from build123d import *

# Parameters (mm, degrees)
SKETCH_1_R          = 4
SKETCH_1_R_2        = 2.95
EXTRUDE_1_DEPTH     = 4.5
SKETCH_1_3_R        = 2.95
SKETCH_1_3_R_2      = 2.5
SKETCH_1_3_R_3      = 1.1
EXTRUDE_2_DEPTH     = 1.7
SKETCH_1_4_R        = 2.95
SKETCH_1_4_R_2      = 2.5
SKETCH_1_4_R_3      = 1.1
CUT_EXTRUDE_1_DEPTH = 0.4
SKETCH_2_R          = 0.6
EXTRUDE_3_DEPTH     = 1.7


with BuildPart() as part:
    # Sketch 1 → Extrude 1 (new body)
    with BuildSketch(Plane.XY):
        Circle(SKETCH_1_R)
        Circle(SKETCH_1_R_2, mode=Mode.SUBTRACT)
    extrude(amount=EXTRUDE_1_DEPTH)

    # Sketch 1_3 → Extrude 2 (add)
    # profile 1 of 2: a face of its own
    with BuildSketch(Plane.XY):
        Circle(SKETCH_1_3_R)
        Circle(SKETCH_1_3_R_2, mode=Mode.SUBTRACT)
    # profile 2 of 2: a face of its own
    with BuildSketch(Plane.XY):
        Circle(SKETCH_1_3_R_2)
        Circle(SKETCH_1_3_R_3, mode=Mode.SUBTRACT)
    extrude(amount=EXTRUDE_2_DEPTH)

    # Sketch 1_4 → Cut-Extrude 1 (cut)
    # profile 1 of 2: a face of its own
    with BuildSketch(Plane.XY):
        Circle(SKETCH_1_4_R)
        Circle(SKETCH_1_4_R_2, mode=Mode.SUBTRACT)
    # profile 2 of 2: a face of its own
    with BuildSketch(Plane.XY):
        Circle(SKETCH_1_4_R_2)
        Circle(SKETCH_1_4_R_3, mode=Mode.SUBTRACT)
    extrude(amount=CUT_EXTRUDE_1_DEPTH, mode=Mode.SUBTRACT)

    # Sketch 2 → Extrude 3 (add)
    with BuildSketch(Plane.XY):
        with BuildLine():
            ThreePointArc((2.491857186, 18.801612903), (0, 21.1), (-2.491857186, 18.801612903))
            Line((-2.491857186, 18.801612903), (-3.986971498, 0.322580645))
            ThreePointArc((-3.986971498, 0.322580645), (0, 4), (3.986971498, 0.322580645))
            Line((3.986971498, 0.322580645), (2.491857186, 18.801612903))
        make_face()
        with Locations((0, 9.801612903)):
            Circle(SKETCH_2_R, mode=Mode.SUBTRACT)
        with Locations((0, 12.801612903)):
            Circle(SKETCH_2_R, mode=Mode.SUBTRACT)
        with Locations((0, 15.801612903)):
            Circle(SKETCH_2_R, mode=Mode.SUBTRACT)
        with Locations((0, 18.801612903)):
            Circle(SKETCH_2_R, mode=Mode.SUBTRACT)
    extrude(amount=EXTRUDE_3_DEPTH)


solid = part.part
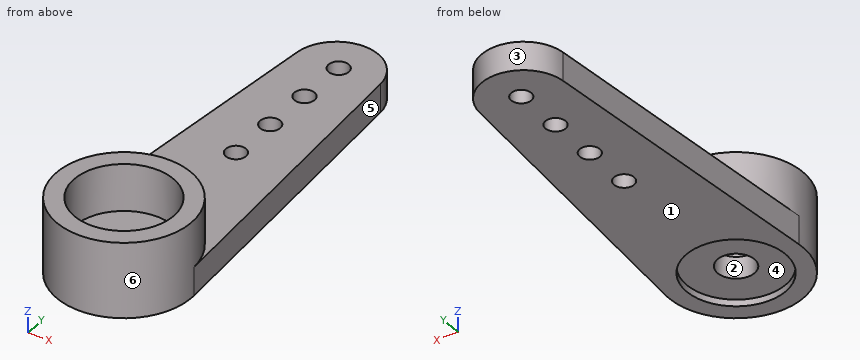
Source: CAD feature listing. Evaluate the final solid. Frame: model axes, mm. Face numbers are marked on the shaded views. A direction names the side the tool comes from. Round coordinates to 2 decimals unless told otherwise and drop trailing zeros. Write each loop counter-clockwise with the first axis right and the second up, starting at its lowest first coordinate (ties: lowest second). Pieces come first, ordered by that corner, then holes. Notation, with made-up numbers: (-4.5, 87) - (46.5, 87) arc R15 ccw to (46.5, 114) - close; hole circle Ø6 at (87, 77.25). An arc over 180 degrees is marked (long way). Use CSV: the item, a comma, the result in double quotes. Start each with the question number.
(1) Material intervals for probe 1 along Z at (x, y) = (-0.25, 17.25); probe 2 along Y at (x, z) = (0, 3.5); probe 3 along Z at (x, y) = (2.25, -1.5), sorted ascending. Write a range as [from, to].
(2) Set-up query: the marked faces 4, 5 and 6. Return all of +Z, -Z, +X, -X, +Y, -Y with unobstructed straight access to the full face (end or side cutting, diameter ignored); none if empty.
(3) Cut plane C-C, the plane z = 1.45. Return loops of the section in (x, y), and give its area (3 significant figures).
(4) Cut plane A-A, the plane y = 0. Return loops of the section in (x, z), and give its area (3 significant figures).
(5) Cut plane D-D, the plane z = 2.55. Return loops of the section in (x, y), and give its area (3 significant figures).
(6) Mould query, pull axis Y, two halves, no side actions, for the marked faces 1, 2 and 3. Classes: pulls with the +Y half, pulls with the -Y half, needs draft (parallel to the pull), parting line crosses it, or undercut.
(7) Cut plane B-B, the plane x = 0. Give the number of separate pieces and of enclosed holes in the cut face, and give its area (3 significant figures).
(8) First-contact query: pin 1 Ø2 at (x, y) = (0.5, 16.5) entering from +Z. Flat tip, straight axial feed; report the tip coordinate or a pass-through.
Geometry says:
1,probe 1,"[0, 1.7]"
1,probe 2,"[-4, -2.95], [2.95, 4]"
1,probe 3,"[0.4, 1.7]"
2,face 4,"-Z"
2,face 5,"+Z, -Z, +X, +Y"
2,face 6,"+Z"
3,outline,"(-3.99, 0.32) arc R4 ccw (long way) to (3.99, 0.32) - (2.49, 18.8) arc R2.5 ccw to (-2.49, 18.8) - close; hole circle Ø2.2 at (0, 0); hole circle Ø1.2 at (0, 9.8); hole circle Ø1.2 at (0, 12.8); hole circle Ø1.2 at (0, 15.8); hole circle Ø1.2 at (0, 18.8)"
3,area,"148 mm²"
4,outline,"(-4, 0) - (-2.95, 0) - (-2.95, 0.4) - (-1.1, 0.4) - (-1.1, 1.7) - (-2.95, 1.7) - (-2.95, 4.5) - (-4, 4.5) - close; (1.1, 0.4) - (2.95, 0.4) - (2.95, 0) - (4, 0) - (4, 4.5) - (2.95, 4.5) - (2.95, 1.7) - (1.1, 1.7) - close"
4,area,"14.3 mm²"
5,outline,"circle Ø8 at (0, 0); hole circle Ø5.9 at (0, 0)"
5,area,"22.9 mm²"
6,face 1,"needs draft"
6,face 2,"undercut"
6,face 3,"pulls with the +Y half"
7,separate pieces,"6"
7,enclosed holes,"0"
7,area,"35.2 mm²"
8,pin 1,"z = 1.7"
